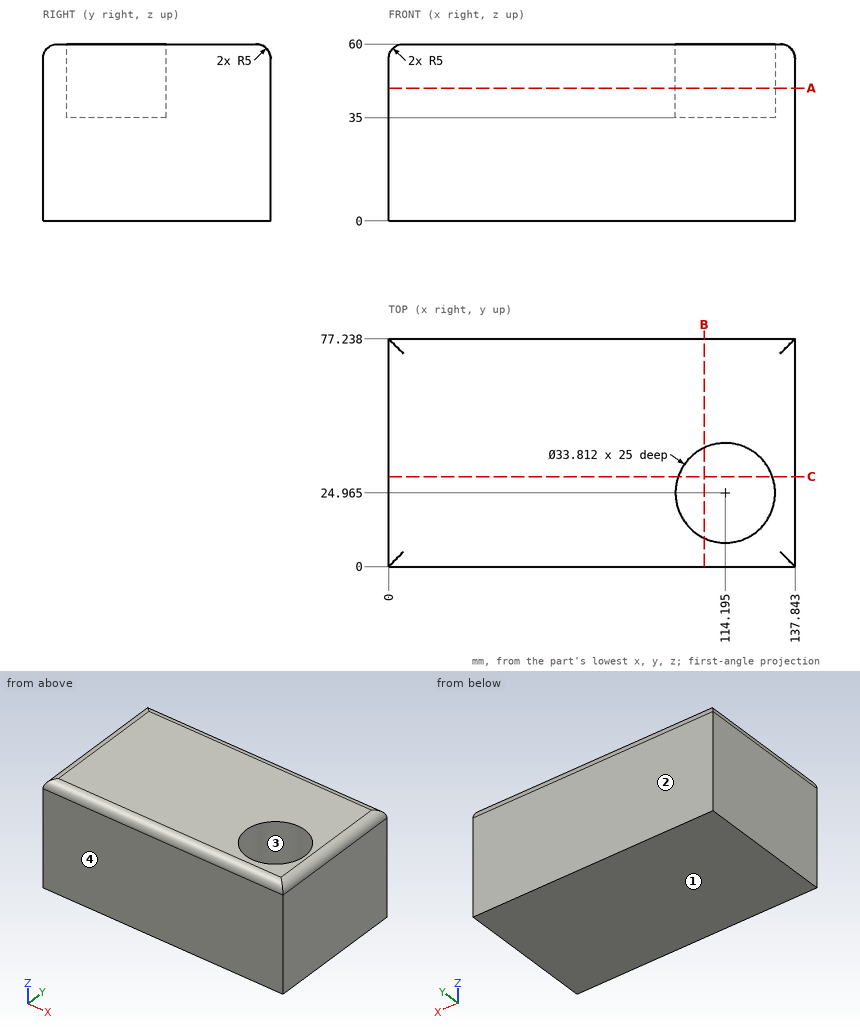
For this review, use the dimensioned drawing (mm, ordinates from the lowest corner) and the shaded views. Coordinates: 2 decimals unless noted, no trailing zeros. Loops run counter-clockwise (first coordinate to the right, second up) from the corner with the lowest first, then second, coordinate; pieces in that order, holes last. Notation, with made-up numbers: M 52.5,-25 L 79.5,-25 A24 ccw 79.5,-3 Z; hole C 31.25,-30 d3. An arc over 180 degrees is marked long. Answer as CSV lines item,"result".
Item 1: Add section A-A on z = 45. State the section outline as (x, y) points (1 decimal), plus the area to 3 significant figures.
Answer list:
outline,"M 0,0 L 137.8,0 L 137.8,77.2 L 0,77.2 Z; hole C 114.2,25 d33.8"
area,"9,750 mm²"
Item 2: For P1, Ø10, axis at x = 110, y = 22.5, coming from the +Z side, flat-tipped, find the tip position at first contact; note if it passes through.
Answer list:
P1,"z = 35"
Item 3: The part is to be moulded in two halves that separate along Y. For the marked faces 1, 2, 3 and 4, say which applies: pulls with the +Y half, pulls with the -Y half, needs draft (parallel to the pull), parting line crosses it, or undercut.
Answer list:
face 1,"needs draft"
face 2,"pulls with the +Y half"
face 3,"undercut"
face 4,"pulls with the -Y half"
Item 4: Add section C-C on y = 30.5. State the section outline as (x, z) points, plus the area to 3 significant figures.
Answer list:
outline,"M 0,0 L 137.84,0 L 137.84,55 A5 ccw 132.84,60 L 130.17,60 L 130.17,35 L 98.22,35 L 98.22,60 L 5,60 A5 ccw 0,55 Z"
area,"7,460 mm²"
Item 5: For probe 1 along X at (y, z) = (34, 40.5) (1 decimal); probe 2 along X at (y, z) = (28.5, 36.5); probe 3 along Y at (x, z) = (129, 55) (1 decimal), list the stretches that pass through material, from the lowest coordinate up.
Answer list:
probe 1,"0 to 99.9, 128.5 to 137.8"
probe 2,"0 to 97.66, 130.73 to 137.84"
probe 3,"0 to 16.8, 33.1 to 77.2"
Item 6: Add section B-B on x = 107. State the section outline as (y, z) points, plus the area to 3 significant figures.
Answer list:
outline,"M 0,0 L 77.24,0 L 77.24,55 A5 ccw 72.24,60 L 40.26,60 L 40.26,35 L 9.67,35 L 9.67,60 L 5,60 A5 ccw 0,55 Z"
area,"3,860 mm²"
